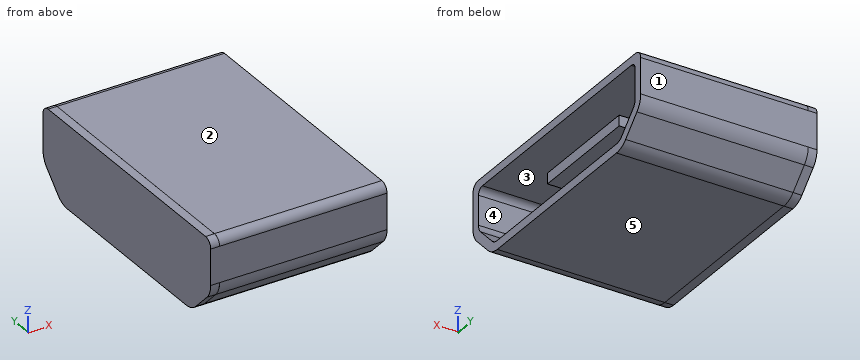
```python
from build123d import *

# Parameters (mm, degrees)
SKETCH077_W                   = 3.25
SKETCH077_H                   = 0.3
PAD102_DEPTH                  = 4
PAD101_DEPTH                  = 0.25
PAD100_DEPTH                  = 4.75
PAD023BODY001_PLACEMENT_ANGLE = 90


with BuildPart() as part:
    # Sketch077 → Pad102 (new body)
    with BuildSketch(Plane(origin=(0, 1.75, 0), x_dir=(-1, 0, 0), z_dir=(0, 1, 0))):
        with Locations((0, 0.5)):
            Rectangle(SKETCH077_W, SKETCH077_H)
    extrude(amount=-PAD102_DEPTH)

    # Sketch076 → Pad101 (join)
    with BuildSketch(Plane.XZ.offset(-1.75)):
        with BuildLine():
            Line((3.565827, 1.174586), (-3.565827, 1.174586))
            ThreePointArc((-3.565827, 1.174586), (-3.731412, 1.105999), (-3.8, 0.940414))
            Line((-3.8, -0.074586), (-3.8, 0.940414))
            ThreePointArc((-3.8, -0.074586), (-3.755291, -0.299355), (-3.62797, -0.489904))
            Line((-3.62797, -0.489904), (-3.115317, -1.002556))
            ThreePointArc((-3.115317, -1.002556), (-2.924768, -1.129877), (-2.7, -1.174586))
            Line((-2.7, -1.174586), (2.7, -1.174586))
            ThreePointArc((2.7, -1.174586), (2.924768, -1.129877), (3.115317, -1.002556))
            Line((3.115317, -1.002556), (3.62797, -0.489904))
            ThreePointArc((3.62797, -0.489904), (3.755291, -0.299355), (3.8, -0.074586))
            Line((3.8, 0.940414), (3.8, -0.074586))
            ThreePointArc((3.8, 0.940414), (3.731412, 1.105999), (3.565827, 1.174586))
        make_face()
    extrude(amount=-PAD101_DEPTH)

    # Sketch078 → Pad100 (join)
    with BuildSketch(Plane(origin=(0, -3, 0), x_dir=(-1, 0, 0), z_dir=(0, 1, 0))):
        with BuildLine():
            Line((-3.565, 1.175), (3.565, 1.175))
            ThreePointArc((3.8, 0.94), (3.73117, 1.10617), (3.565, 1.175))
            Line((3.8, 0.94), (3.8, -0.075))
            ThreePointArc((3.62797, -0.490317), (3.755291, -0.299768), (3.8, -0.075))
            Line((3.62797, -0.490317), (3.115317, -1.00297))
            ThreePointArc((2.7, -1.175), (2.924768, -1.130291), (3.115317, -1.00297))
            Line((2.7, -1.175), (-2.7, -1.175))
            ThreePointArc((-3.115317, -1.00297), (-2.924768, -1.130291), (-2.7, -1.175))
            Line((-3.115317, -1.00297), (-3.62797, -0.490317))
            ThreePointArc((-3.8, -0.075), (-3.755291, -0.299768), (-3.62797, -0.490317))
            Line((-3.8, -0.075), (-3.8, 0.94))
            ThreePointArc((-3.565, 1.175), (-3.73117, 1.10617), (-3.8, 0.94))
        make_face()
        with BuildLine():
            Line((-3.373361, 0.935), (3.373361, 0.935))
            ThreePointArc((3.55, 0.758361), (3.498264, 0.883264), (3.373361, 0.935))
            Line((3.55, 0.758361), (3.55, -0.077967))
            ThreePointArc((3.453274, -0.311484), (3.524862, -0.204346), (3.55, -0.077967))
            Line((3.453274, -0.311484), (2.936484, -0.828274))
            ThreePointArc((2.702967, -0.925), (2.829346, -0.899862), (2.936484, -0.828274))
            Line((2.702967, -0.925), (-2.702967, -0.925))
            ThreePointArc((-2.936484, -0.828274), (-2.829346, -0.899862), (-2.702967, -0.925))
            Line((-2.936484, -0.828274), (-3.453274, -0.311484))
            ThreePointArc((-3.55, -0.077967), (-3.524862, -0.204346), (-3.453274, -0.311484))
            Line((-3.55, -0.077967), (-3.55, 0.758361))
            ThreePointArc((-3.373361, 0.935), (-3.498264, 0.883264), (-3.55, 0.758361))
        make_face(mode=Mode.SUBTRACT)
    extrude(amount=PAD100_DEPTH)


with BuildPart() as part_1:
    # Pad023Body001 placement: moved
    add(part.part.moved(Location((15, -6.7, 1.175))).rotate(Axis((15, -6.7, 1.175), (0, 0, 1)), PAD023BODY001_PLACEMENT_ANGLE))


solid = part_1.part
```
Design review of the part built by this model. Coordinates are the model's own, in mm. Face numbers are marked on the shaded views. A direction names the side the tool comes from. Coordinates: 2 decimals unless noted, no trailing zeros. Order: outer loops, then holes, each group sorted by start corner. A loop starts at its lowest first (then second) coordinate and runs counter-clockwise, first axis right, second up. Notation, with made-up numbers: (-8.75, 59) - (23.25, 59) arc R26 cw to (23.25, 89) - close; hole circle Ø6 at (-7.75, 26). An arc over 180 degrees is marked (long way). Answer in a Markdown table with one row per item.
(1) Clearance check with a flat-ended pin moving along its axis: pin 1 (0.9 mm diameter, centred on y = -7, z = 1.5, fed in from +X). State where the tip first meets the part, or that it passes through.
Checked values:
| item | result |
|---|---|
| pin 1 | x = 17.25 |
(2) The part is to be moulded in two halves that separate along Y. For the marked faces 1, 2 and 3, say which applies: released by +Y, released by -Y, zero draft, split by the parting line, or undercut.
Checked values:
| item | result |
|---|---|
| face 1 | released by +Y |
| face 2 | zero draft |
| face 3 | undercut |
(3) Consider section A-A on x = 13.65. State the section outline as (y, z) points (3 decimals).
Checked values:
| item | result |
|---|---|
| outline | (-10.5, 1.1) arc R0.587 ccw to (-10.328, 0.685) - (-9.815, 0.172) arc R0.587 ccw to (-9.4, 0) - (-4, 0) arc R0.587 ccw to (-3.585, 0.172) - (-3.072, 0.685) arc R0.587 ccw to (-2.9, 1.1) - (-2.9, 2.115) arc R0.235 ccw to (-3.135, 2.35) - (-10.265, 2.35) arc R0.235 ccw to (-10.5, 2.115) - close; (-8.325, 1.525) - (-5.075, 1.525) - (-5.075, 1.825) - (-8.325, 1.825) - close; hole (-10.25, 1.097) arc R0.33 ccw to (-10.153, 0.864) - (-9.636, 0.347) arc R0.33 ccw to (-9.403, 0.25) - (-3.997, 0.25) arc R0.33 ccw to (-3.764, 0.347) - (-3.247, 0.864) arc R0.33 ccw to (-3.15, 1.097) - (-3.15, 1.933) arc R0.177 ccw to (-3.327, 2.11) - (-10.073, 2.11) arc R0.177 ccw to (-10.25, 1.933) - close |
(4) For the marked faces 4 and 5, list the 3-axis set-ups (+Z, -Z, +X, -X, +Y, -Y) from which the entire face can be reached by the end or side of a thin tool; tool diameter is ignored.
Checked values:
| item | result |
|---|---|
| face 4 | +X |
| face 5 | -Z, +X, -X, +Y, -Y |
(5) Consider section C-C on z = 1.7. State the section outline as (x, y) points (3 decimals), plus the area to 3 significant figures.
Checked values:
| item | result |
|---|---|
| outline | (13, -10.5) - (18, -10.5) - (18, -10.25) - (13.25, -10.25) - (13.25, -8.325) - (17.25, -8.325) - (17.25, -5.075) - (13.25, -5.075) - (13.25, -3.15) - (18, -3.15) - (18, -2.9) - (13, -2.9) - close |
| area | 17.3 mm^2 |
(6) Wall thickness on line 1 along Z through (x, y) = (16.2, -6.25) (3 decimals); line 2 along Z through (x, y) = (13.65, -8.75); line 3 along Y through (x, z) = (17.25, 1.4): over which ranges is each line inside the solid? List them lowest first. Write a range as from..to.
Checked values:
| item | result |
|---|---|
| line 1 | 0..0.25, 1.525..1.825, 2.11..2.35 |
| line 2 | 0..0.25, 2.11..2.35 |
| line 3 | -10.5..-10.25, -3.15..-2.9 |
